from build123d import *

# Parameters (mm, degrees)
SKETCH1_W           = 50
SKETCH1_H           = 155
BOSS_EXTRUDE1_DEPTH = 2
SKETCH2_W           = 50
SKETCH2_H           = 2
BOSS_EXTRUDE2_DEPTH = 50
SKETCH3_W           = 50
SKETCH3_H           = 2
BOSS_EXTRUDE3_DEPTH = 50
SKETCH4_R           = 2
CUT_EXTRUDE1_DEPTH  = 145.97586006
SKETCH5_R           = 5
CUT_EXTRUDE2_DEPTH  = 103.732662771
SKETCH6_R           = 1.5
CUT_EXTRUDE3_DEPTH  = 102.084123382
SKETCH7_W           = 50
SKETCH7_H           = 2
BOSS_EXTRUDE4_DEPTH = 50
CUT_EXTRUDE5_REACH  = 129.769
SKETCH9_R           = 11.5
SKETCH9_R_2         = 1.5
BOSS_EXTRUDE5_DEPTH = 2
BOSS_EXTRUDE6_DEPTH = 20


with BuildPart() as part:
    # Sketch1 → Boss-Extrude1 (new body)
    with BuildSketch(Plane.XY):
        Rectangle(SKETCH1_W, SKETCH1_H)
    extrude(amount=BOSS_EXTRUDE1_DEPTH)

    # Sketch2 → Boss-Extrude2 (add)
    with BuildSketch(Plane.XY.offset(2)):
        with Locations((0, -56.5)):
            Rectangle(SKETCH2_W, SKETCH2_H)
    extrude(amount=BOSS_EXTRUDE2_DEPTH)

    # Sketch3 → Boss-Extrude3 (add)
    with BuildSketch(Plane.XY.offset(2)):
        with Locations((0, 6.5)):
            Rectangle(SKETCH3_W, SKETCH3_H)
    extrude(amount=BOSS_EXTRUDE3_DEPTH)

    # Sketch4 → Cut-Extrude1 (cut, through all)
    with BuildSketch(Plane(origin=(0, -55.5, 0), x_dir=(1, 0, 0), z_dir=(0, 1, 0))):
        with Locations(Location((-16.970562748, -43.970562748, 0), (0, 0, 270))):
            Circle(SKETCH4_R)
        with Locations(Location((16.970562748, -43.970562748, 0), (0, 0, 270))):
            Circle(SKETCH4_R)
        with Locations(Location((16.970562748, -10.029437252, 0), (0, 0, 270))):
            Circle(SKETCH4_R)
        with Locations(Location((-16.970562748, -10.029437252, 0), (0, 0, 270))):
            Circle(SKETCH4_R)
    extrude(amount=-CUT_EXTRUDE1_DEPTH, mode=Mode.SUBTRACT)

    # Sketch5 → Cut-Extrude2 (cut, through all)
    with BuildSketch(Plane(origin=(0, 7.5, 0), x_dir=(1, 0, 0), z_dir=(0, 1, 0))):
        with Locations(Location((0, -27, 0), (0, 0, 270))):
            Circle(SKETCH5_R)
    extrude(amount=-CUT_EXTRUDE2_DEPTH, mode=Mode.SUBTRACT)

    # Sketch6 → Cut-Extrude3 (cut, through all)
    with BuildSketch(Plane.XZ.offset(-5.5)):
        with Locations((0, 41)):
            Circle(SKETCH6_R)
        with Locations((14, 27)):
            Circle(SKETCH6_R)
        with Locations((0, 13)):
            Circle(SKETCH6_R)
        with Locations((-14, 27)):
            Circle(SKETCH6_R)
    extrude(amount=-CUT_EXTRUDE3_DEPTH, mode=Mode.SUBTRACT)

    # Sketch7 → Boss-Extrude4 (add)
    with BuildSketch(Plane.XY.offset(2)):
        with Locations((0, 35.5)):
            Rectangle(SKETCH7_W, SKETCH7_H)
    extrude(amount=BOSS_EXTRUDE4_DEPTH)

    # Sketch9 → Cut-Extrude5 (cut, up to next)
    with BuildSketch(Plane(origin=(0, 36.5, 0), x_dir=(1, 0, 0), z_dir=(0, 1, 0)), mode=Mode.PRIVATE) as cut_extrude5_sk1:
        with Locations(Location((0, -27, 0), (0, 0, 270))):
            Circle(SKETCH9_R)
    cut_extrude5_tool1 = extrude(cut_extrude5_sk1.sketch, amount=-CUT_EXTRUDE5_REACH, mode=Mode.PRIVATE) & part.part
    # Sketch9 → Cut-Extrude5 (cut, up to next)
    with BuildSketch(Plane(origin=(0, 36.5, 0), x_dir=(1, 0, 0), z_dir=(0, 1, 0)), mode=Mode.PRIVATE) as cut_extrude5_sk2:
        with Locations((-14, -27)):
            Circle(SKETCH9_R_2)
    cut_extrude5_tool2 = extrude(cut_extrude5_sk2.sketch, amount=-CUT_EXTRUDE5_REACH, mode=Mode.PRIVATE) & part.part
    # Sketch9 → Cut-Extrude5 (cut, up to next)
    with BuildSketch(Plane(origin=(0, 36.5, 0), x_dir=(1, 0, 0), z_dir=(0, 1, 0)), mode=Mode.PRIVATE) as cut_extrude5_sk3:
        with Locations((0, -41)):
            Circle(SKETCH9_R_2)
    cut_extrude5_tool3 = extrude(cut_extrude5_sk3.sketch, amount=-CUT_EXTRUDE5_REACH, mode=Mode.PRIVATE) & part.part
    # Sketch9 → Cut-Extrude5 (cut, up to next)
    with BuildSketch(Plane(origin=(0, 36.5, 0), x_dir=(1, 0, 0), z_dir=(0, 1, 0)), mode=Mode.PRIVATE) as cut_extrude5_sk4:
        with Locations((14, -27)):
            Circle(SKETCH9_R_2)
    cut_extrude5_tool4 = extrude(cut_extrude5_sk4.sketch, amount=-CUT_EXTRUDE5_REACH, mode=Mode.PRIVATE) & part.part
    # Sketch9 → Cut-Extrude5 (cut, up to next)
    with BuildSketch(Plane(origin=(0, 36.5, 0), x_dir=(1, 0, 0), z_dir=(0, 1, 0)), mode=Mode.PRIVATE) as cut_extrude5_sk5:
        with Locations((0, -13)):
            Circle(SKETCH9_R_2)
    cut_extrude5_tool5 = extrude(cut_extrude5_sk5.sketch, amount=-CUT_EXTRUDE5_REACH, mode=Mode.PRIVATE) & part.part
    add(cut_extrude5_tool1.solids().sort_by_distance((0, 36.5, 27))[0], mode=Mode.SUBTRACT)
    add(cut_extrude5_tool2.solids().sort_by_distance((-14, 36.5, 27))[0], mode=Mode.SUBTRACT)
    add(cut_extrude5_tool3.solids().sort_by_distance((0, 36.5, 41))[0], mode=Mode.SUBTRACT)
    add(cut_extrude5_tool4.solids().sort_by_distance((14, 36.5, 27))[0], mode=Mode.SUBTRACT)
    add(cut_extrude5_tool5.solids().sort_by_distance((0, 36.5, 13))[0], mode=Mode.SUBTRACT)

    # Sketch12 → Boss-Extrude5 (add)
    with BuildSketch(Plane.ZY.offset(25)):
        Polygon((2, 65.367513459), (52, 36.5), (2, 36.5), align=None)
        Polygon((2, -77.5), (2, -57.5), (52, -57.5), align=None)
        Polygon((2, 34.5), (52, 34.5), (2, 7.5), align=None)
    boss_extrude5 = extrude(amount=-BOSS_EXTRUDE5_DEPTH)

    # Mirror1: Boss-Extrude5 across plane
    add(boss_extrude5.mirror(Plane(origin=(0, 0, 0), x_dir=(0, 0, 1), z_dir=(1, 0, 0))))

    # Sketch13 → Boss-Extrude6 (add)
    with BuildSketch(Plane(origin=(0, 0, 0), x_dir=(-1, 0, 0), z_dir=(0, 0, -1))):
        Polygon((-25, 58.5), (25, 58.5), (25, 56.5), (1, 56.5), (1, -56.5), (25, -56.5), (25, -58.5), (-25, -58.5), (-25, -56.5), (-1, -56.5), (-1, 56.5), (-25, 56.5), align=None)
    extrude(amount=BOSS_EXTRUDE6_DEPTH)


solid = part.part
Model file for the job. Use its own axes, mm. A direction names the side the tool comes from. Give positions to 0.01 mm unless a question says otherwise; leave off trailing zeros. Order: outer loops, then holes, each group sorted by start corner. A loop starts at its lowest first (then second) coordinate and runs counter-clockwise, first axis right, second up. Notation, with made-up numbers: (22, 30) -> (57, 30) arc R14 ccw to (57, 38) -> close; hole circle Ø4 at (-33.5, 85). An arc over 180 degrees is marked (long way). Use CSV: the item, a comma, the result in double quotes.
1. Drop flat-ended pins along their axis: pin 1 (19 mm diameter, centred on x = -16.5, y = 12, fed in from -Z); pin 2 (16 mm diameter, centred on x = 0, z = 27, fed in from -Y); pin 3 (6 mm diameter, centred on y = -2, z = -8, fed in from -X). Give the stop position or say it passes through.
Outcome:
pin 1,"z = 0"
pin 2,"y = -57.5"
pin 3,"x = -1"
2. Band-saw the part on D-D, the plane z = 27. Count the separate pieces of the cut face and the enclosed holes in it, then the cut area to 3 significant figures.
Outcome:
separate pieces,"10"
enclosed holes,"0"
area,"342 mm²"
3. Drill centre lines: line 1 along Y through (x, z) = (19, 28); line 2 along X through (y, z) = (35, 27); line 3 along Y through (x, z) = (21.5, -12). Where is each one in solid material? Low to high. Write a range as from..to.
Outcome:
line 1,"-57.5..-55.5, 5.5..7.5, 34.5..36.5"
line 2,"-25..-15.5, -12.5..-11.5, 11.5..12.5, 15.5..25"
line 3,"-58.5..-56.5, 56.5..58.5"
4. Band-saw the part on B-B, the plane z = -4.5. Give the cut face in (x, y).
Outcome:
outline,"(-25, -58.5) -> (25, -58.5) -> (25, -56.5) -> (1, -56.5) -> (1, 56.5) -> (25, 56.5) -> (25, 58.5) -> (-25, 58.5) -> (-25, 56.5) -> (-1, 56.5) -> (-1, -56.5) -> (-25, -56.5) -> close"
5. Mould opens along X. For faces 6 (the flat face through (13, -56.5, -10)), 7 (the flat face through (-1, 1, -10)), 8 (the cylindrical face through (0, 7, 22)) say: +X half, -X half, draft (parallel to the pull), parting line (faces both ways), or undercut.
Outcome:
face 6,"draft"
face 7,"-X half"
face 8,"undercut"
6. 3-axis set-ups, long thin cutter, end or side, ignore diameter. For faces 1 (the flat face through (-23, -63, 16)), 2 (the flat face through (-13, 56.5, -10)), 3 (the flat face through (-11, 36.5, 21)), 4 (the flat face through (-11, 34.5, 21)), 5 (the flat face through (0, 68, 0)): which of +Z, -Z, +X, -X, +Y, -Y reach the whole face in a straight line?
Outcome:
face 1,"+Z, -Y"
face 2,"-Z, -X"
face 3,"+Z, +Y"
face 4,"+Z"
face 5,"-Z, +X, -X, +Y"
7. Band-saw the part on C-C, the plane z = 19.5. Give the cut face in (x, y), then the cut area to 3 significant figures.
Outcome:
outline,"(-25, -70.5) -> (-23, -70.5) -> (-23, -57.5) -> (23, -57.5) -> (23, -70.5) -> (25, -70.5) -> (25, -55.5) -> (-25, -55.5) -> close; (-25, 5.5) -> (25, 5.5) -> (25, 7.5) -> (-25, 7.5) -> close; (-25, 16.95) -> (-23, 16.95) -> (-23, 34.5) -> (-8.72, 34.5) -> (-8.72, 36.5) -> (-23, 36.5) -> (-23, 55.26) -> (-25, 55.26) -> close; (8.72, 34.5) -> (23, 34.5) -> (23, 16.95) -> (25, 16.95) -> (25, 55.26) -> (23, 55.26) -> (23, 36.5) -> (8.72, 36.5) -> close"
area,"462 mm²"
8. Band-saw the part on A-A, the plane y = -40. Give the cut face in (x, z), then the cut area to 3 significant figures.
Outcome:
outline,"(-25, 0) -> (-1, 0) -> (-1, -20) -> (1, -20) -> (1, 0) -> (25, 0) -> (25, 2) -> (-25, 2) -> close"
area,"140 mm²"
